from build123d import *

# Parameters (mm, degrees)
SKETCH1_R           = 18.5
SKETCH1_R_2         = 1.5
SKETCH1_R_3         = 6.1
BOSS_EXTRUDE1_DEPTH = 12
SKETCH2_R           = 18
BOSS_EXTRUDE2_DEPTH = 50
SKETCH3_R           = 3
BOSS_EXTRUDE3_DEPTH = 21
SKETCH4_R           = 6.1
BOSS_EXTRUDE4_DEPTH = 12
CUT_EXTRUDE1_START  = -5
CUT_EXTRUDE1_DEPTH  = 5
SCALE1_SCALE        = 0.8
SCALE3_SCALE        = 1.1


with BuildPart() as part:
    # Sketch1 → Boss-Extrude1 (new body)
    with BuildSketch(Plane.XY):
        with Locations((6.10211523, 32.843167441)):
            Circle(SKETCH1_R)
        with Locations((21.60211523, 32.843167441)):
            Circle(SKETCH1_R_2, mode=Mode.SUBTRACT)
        with Locations((13.85211523, 19.419773682)):
            Circle(SKETCH1_R_2, mode=Mode.SUBTRACT)
        with Locations((-1.64788477, 19.419773682)):
            Circle(SKETCH1_R_2, mode=Mode.SUBTRACT)
        with Locations((-9.39788477, 32.843167441)):
            Circle(SKETCH1_R_2, mode=Mode.SUBTRACT)
        with Locations((-1.64788477, 46.266561199)):
            Circle(SKETCH1_R_2, mode=Mode.SUBTRACT)
        with Locations((13.85211523, 46.266561199)):
            Circle(SKETCH1_R_2, mode=Mode.SUBTRACT)
        with Locations((6.10211523, 40.343167441)):
            Circle(SKETCH1_R_3, mode=Mode.SUBTRACT)
    extrude(amount=BOSS_EXTRUDE1_DEPTH)

    # Sketch2 → Boss-Extrude2 (add)
    with BuildSketch(Plane(origin=(0, 0, 0), x_dir=(-1, 0, 0), z_dir=(0, 0, -1))):
        with Locations((-6.10211523, 32.843167441)):
            Circle(SKETCH2_R)
    extrude(amount=BOSS_EXTRUDE2_DEPTH)



with BuildPart() as body_2:
    # Sketch3 → Boss-Extrude3 (new body)
    with BuildSketch(Plane.XY.offset(12)):
        with Locations(Location((6.10211523, 40.343167441, 0), (0, 0, 180))):
            Circle(SKETCH3_R)
    extrude(amount=BOSS_EXTRUDE3_DEPTH)


with BuildPart() as part_1:
    add(part.part)

    add(body_2.part)  # Boss-Extrude4 merges body 2
    # Sketch4 → Boss-Extrude4 (add)
    with BuildSketch(Plane.XY):
        with Locations((6.10211523, 40.343167441)):
            Circle(SKETCH4_R)
    extrude(amount=BOSS_EXTRUDE4_DEPTH)

    # Sketch5 → Cut-Extrude1 (cut)
    with BuildSketch(Plane.XY.offset(12).offset(CUT_EXTRUDE1_START)):
        with BuildLine():
            Line((6.10211523, 50.343167441), (6.10211523, 51.343167441))
            ThreePointArc((6.10211523, 51.343167441), (3.060733965, 51.091455031), (0.10211523, 50.343167441))
            Line((0.10211523, 50.343167441), (6.10211523, 50.343167441))
        make_face()
        with BuildLine():
            ThreePointArc((12.10211523, 50.343167441), (9.143496496, 51.091455031), (6.10211523, 51.343167441))
            Line((6.10211523, 51.343167441), (6.10211523, 50.343167441))
            Line((6.10211523, 50.343167441), (12.10211523, 50.343167441))
        make_face()
    extrude(amount=CUT_EXTRUDE1_DEPTH, mode=Mode.SUBTRACT)


with BuildPart() as part_2:
    # Scale1: scaled about (6.10211523, 32.901644157, -18.561855602)
    add(part_1.part.scale(SCALE1_SCALE).moved(Location((1.220423046, 6.580328831, -3.71237112))))


with BuildPart() as part_3:
    # Scale3: scaled about (6.10211523, 32.901644157, -18.561855602)
    add(part_2.part.scale(SCALE3_SCALE).moved(Location((-0.610211523, -3.290164416, 1.85618556))))


solid = part_3.part
Verification items for the finished model (mm, model axes). A direction names the side the tool comes from. Give positions to 0.01 mm unless a question says otherwise; leave off trailing zeros. Write each loop counter-clockwise with the first axis right and the second up, starting at its lowest first coordinate (ties: lowest second). Pieces come first, ordered by that corner, then holes.
(1) Access from +Z, -Z, +X, -X, +Y, -Y to the whole of each face (thin tool, end or side, straight path). Record for faces 1 (the face through (2.57, 16.96, 2.98)), 2 (the face through (6, 48.25, 6)), 3 (the face through (8.164, 48.555, -23.919)), 4 (the face through (20, 33, -2.227)), 5 (the face through (6, 33, -46.227)).
(2) Gauge pin test, flat ends, axial feed: pin 1 (3.5 mm diameter, centred on x = 7, z = 6.5, fed in from +Y); pin 2 (12 mm diameter, centred on x = -6.5, z = 4, fed in from +Y); pin 3 (2 mm diameter, centred on x = -1, y = 44, fed in from +Z); pin 4 (6 mm diameter, centred on x = 6.5, z = 2.5, fed in from +Y). Record the tip position at first contact, or that the pin passes through.
(3) Cross-section at B-B (x = 7.5). Enter the section's corners in (y, z).
(4) Cross-section at C-C (z = 18.5). Enter the section's corners in (x, y), plus the area to 3 significant figures.
(5) Cross-section at D-D (x = 2.5). Enter the section's corners in (y, z), plus the area to 3 significant figures.
(6) Material ranges on line 1 (Z direction, x = -3, y = 20); line 2 (X direction, y = 28, z = -37.5); line 3 (X direction, y = 37.5, z = -1.5), recorded low to high.
(7) Cross-section at A-A (y = 38). Enter the section's corners in (x, z).
Worked out:
1. face 1: +Z, -Z
1. face 2: +Z, +X, -X, +Y
1. face 3: -Z
1. face 4: +Z
1. face 5: -Z, +X, -X, +Y, -Y
2. pin 1: stops at y = 48.25
2. pin 2: stops at y = 47.73
2. pin 3: stops at z = 8.33
2. pin 4: stops at y = 49.13
3. outline: (16.63, -2.23) - (17.07, -2.23) - (17.07, -46.23) - (48.63, -46.23) - (48.63, -2.23) - (49.07, -2.23) - (49.07, 3.93) - (48.25, 3.93) - (48.25, 8.33) - (41.69, 8.33) - (41.69, 26.81) - (37.21, 26.81) - (37.21, 8.33) - (16.63, 8.33) - close
4. outline: circle Ø5.28 at (6.1, 39.45)
4. area: 21.9 mm2
5. outline: (16.97, -2.23) - (17.43, -2.23) - (17.43, -46.23) - (48.28, -46.23) - (48.28, -2.23) - (48.73, -2.23) - (48.73, 3.93) - (48.25, 3.93) - (48.25, 8.33) - (16.97, 8.33) - close
5. area: 1,690 mm2
6. line 1: z = -46.23 to 8.33
6. line 2: x = -8.98 to 21.18
6. line 3: x = -9.5 to 21.7
7. outline: (-9.34, -2.23) - (-8.88, -2.23) - (-8.88, -46.23) - (21.08, -46.23) - (21.08, -2.23) - (21.55, -2.23) - (21.55, 8.33) - (8.31, 8.33) - (8.31, 26.81) - (3.9, 26.81) - (3.9, 8.33) - (-9.34, 8.33) - close
